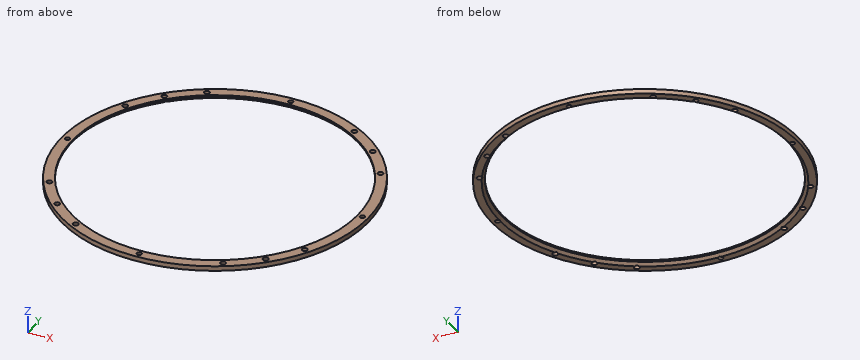
```python
from build123d import *

# Parameters (mm, degrees)
F_4_5_4_5_DIAMETER_HOLE1_D = 4.5
CIRPATTERN1_COUNT          = 12
F_4_0_4_DIAMETER_HOLE1_D   = 4
CIRPATTERN2_COUNT          = 4
F_4_5_4_5_DIAMETER_HOLE2_D = 4.5
CIRPATTERN3_COUNT          = 4


with BuildPart() as part:
    # Sketch1 → Revolve1 (revolve)
    with BuildSketch(Plane(origin=(0, 0, 0), x_dir=(0, 0, -1), z_dir=(1, 0, 0)), mode=Mode.PRIVATE) as revolve1_sk:
        Polygon((0, 122.55), (-2.5, 120.05), (-4, 120.05), (-4, 129), (0, 129), align=None)
    revolve(revolve1_sk.sketch.rotate(Axis((0, 0, 27.349424097), (0, 0, -1)), 90), axis=Axis((0, 0, 27.349424097), (0, 0, -1)))  # turned: the seam where the file's is

    # Ø4.5 (4.5) Diameter Hole1 (through all)
    with Locations(Plane.XY.offset(4)):
        with Locations((62.125, 107.60365642)):
            f_4_5_4_5_diameter_hole1 = Hole(F_4_5_4_5_DIAMETER_HOLE1_D / 2)

    # CirPattern1: Ø4.5 (4.5) Diameter Hole1 ×12 about axis, 4 skipped
    cirpattern1_axis = Axis((0, 0, -80.9), (0, 0, 1))
    add([f_4_5_4_5_diameter_hole1.rotate(cirpattern1_axis, i * 360 / CIRPATTERN1_COUNT) for i in range(1, CIRPATTERN1_COUNT) if i not in (1, 4, 7, 10)], mode=Mode.SUBTRACT)

    # Ø4.0 (4) Diameter Hole1 (through all)
    with Locations(Plane.XY.offset(4)):
        with Locations((124.25, 0)):
            f_4_0_4_diameter_hole1 = Hole(F_4_0_4_DIAMETER_HOLE1_D / 2)

    # CirPattern2: Ø4.0 (4) Diameter Hole1 ×4 about axis
    cirpattern2_axis = Axis((0, 0, 0), (0, 0, 1))
    for i in range(1, CIRPATTERN2_COUNT):
        add(f_4_0_4_diameter_hole1.rotate(cirpattern2_axis, i * 360 / CIRPATTERN2_COUNT), mode=Mode.SUBTRACT)

    # Ø4.5 (4.5) Diameter Hole2 (through all)
    with Locations(Plane.XY.offset(4)):
        with Locations((87.858017562, 87.858017562)):
            f_4_5_4_5_diameter_hole2 = Hole(F_4_5_4_5_DIAMETER_HOLE2_D / 2)

    # CirPattern3: Ø4.5 (4.5) Diameter Hole2 ×4 about axis
    cirpattern3_axis = Axis((0, 0, 0), (0, 0, 1))
    for i in range(1, CIRPATTERN3_COUNT):
        add(f_4_5_4_5_diameter_hole2.rotate(cirpattern3_axis, i * 360 / CIRPATTERN3_COUNT), mode=Mode.SUBTRACT)


solid = part.part
```
The model under review builds one solid part; all positions refer to its coordinate system, in mm. Coordinates: 2 decimals unless noted, no trailing zeros. Answer as CSV lines item,"result".
Item 1: For L1, parallel to Y at x = 89, z = 0.7; L2, parallel to Y at x = -106.5, z = 3.6; L3, parallel to X at y = 49, z = 1.5, list the stretches that pass through material, from the lowest coordinate up.
Results below:
L1,"y = -93.38 to -89.8, -85.92 to -83.23, 83.23 to 85.92, 89.8 to 93.38"
L2,"y = -72.79 to -64.09, -60.16 to -55.41, 55.41 to 60.16, 64.09 to 72.79"
L3,"x = -119.33 to -110.69, 110.69 to 119.33"
Item 2: Take a section at A-A, the plane z = 1.85. Count the separate pieces of the cut face and the enclosed holes in it, and give its area (3 significant figures).
Results below:
separate pieces,"1"
enclosed holes,"17"
area,"6,270 mm2"
Item 3: Insertion check: pin 1 (1 mm diameter, centred on x = -66.5, z = 2.5, fed in from +Y); pin 2 (2 mm diameter, centred on y = 96.5, z = 2.5, fed in from -X); pin 3 (2 mm diameter, centred on y = 75.5, z = 1.5, fed in from +X). Each pin has a flat end and moves straight along its axis. Give the tip position at first contact, or say it passes through.
Results below:
pin 1,"stops at y = 110.84"
pin 2,"stops at x = -86.72"
pin 3,"stops at x = 105.31"
